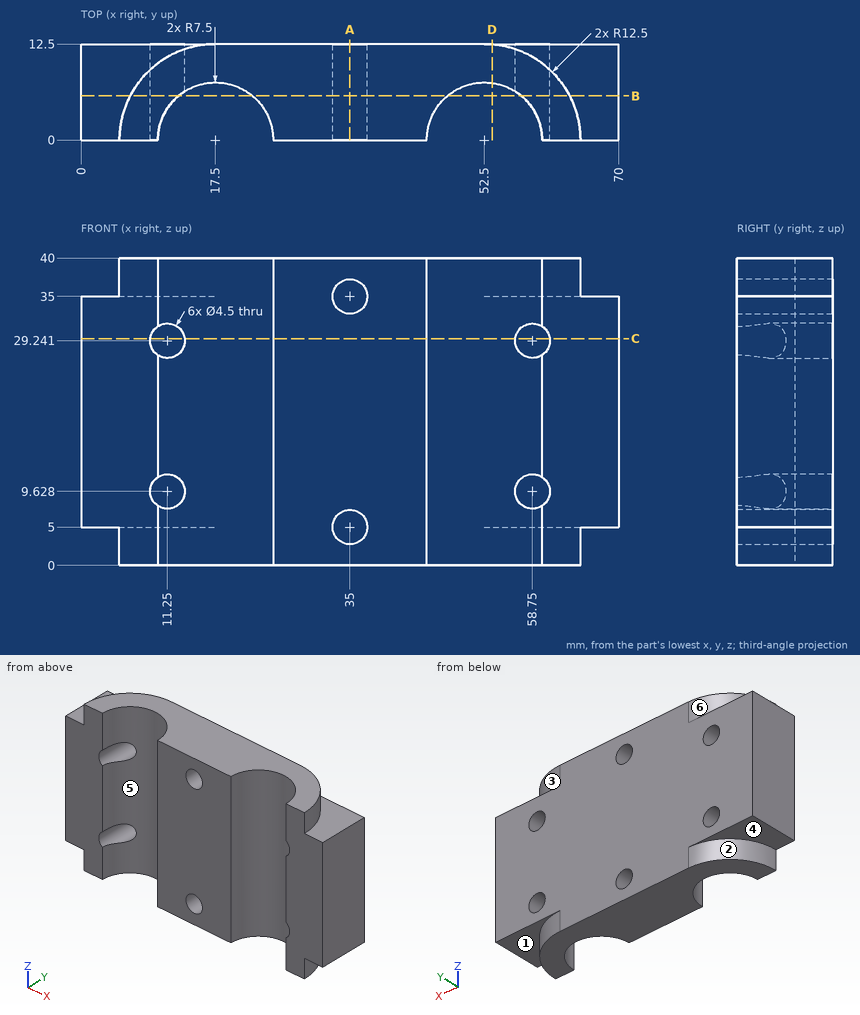
Check sheet for the drawn part. Datum: minimum x, y, z corner. Units: mm. A direction names the side the tool comes from. Give positions to 0.01 mm unless a question says otherwise; leave off trailing zeros. Loops run counter-clockwise (first coordinate to the right, second up) from the corner with the lowest first, then second, coordinate; pieces in that order, holes last.
1) Thickness scan on line 1 along Z through (x, y) = (11.25, 4.5); line 2 along X through (y, z) = (6, 17); line 3 along X through (y, z) = (1.5, 8.5). Record the ranges inside material, lowest first.
2) Set-up check for the marked faces 1, 2 and 3: record each of +Z, -Z, +X, -X, +Y, -Y from which the full face is reachable in a straight line by a thin tool's end or side.
3) Depth check by flat-ended pin: pin 1 Ø4 at (x, z) = (35, 5) entering from +Y. Enter the tip coordinate at first touch or a pass-through.
4) Sectioned sample at C-C, the plane z = 29.5. Enter the section's corners in (x, y) (1 decimal).
5) Sectioned sample at A-A, the plane x = 35. Enter the section's corners in (y, z).
6) Draft check along X on the marked faces 4, 5 and 6. Enter one of: pulls with the +X half, pulls with the -X half, needs draft (parallel to the pull), parting line crosses it, or undercut.
7) Sectioned sample at B-B, the plane y = 5.75. Count the separate pieces of the cut face and the enclosed holes in it, then the cut area to 3 significant figures.
8) Sectioned sample at D-D, the plane x = 53.5. Enter the section's corners in (y, z), then the cut area to 3 significant figures.
Answers:
1. line 1: z = 0 to 7.38, 11.88 to 26.99, 31.49 to 40
1. line 2: x = 0 to 13, 22 to 48, 57 to 70
1. line 3: x = 0 to 9.3, 24.85 to 45.15, 60.7 to 70
2. face 1: -Z, +X, +Y
2. face 2: -Z, -X, +Y
2. face 3: +Z, +X, +Y
3. pin 1: passes through
4. outline: (0, 0) - (9, 0) - (9, 12.5) - (0, 12.5) - close; (13.5, 6.3) arc R7.5 cw to (25, 0) - (45, 0) arc R7.5 cw to (56.5, 6.3) - (56.5, 12.5) - (13.5, 12.5) - close; (61, 0) - (70, 0) - (70, 12.5) - (61, 12.5) - close
5. outline: (0, 0) - (12.5, 0) - (12.5, 2.75) - (0, 2.75) - close; (0, 7.25) - (12.5, 7.25) - (12.5, 32.75) - (0, 32.75) - close; (0, 37.25) - (12.5, 37.25) - (12.5, 40) - (0, 40) - close
6. face 4: needs draft
6. face 5: undercut
6. face 6: pulls with the -X half
7. separate pieces: 3
7. enclosed holes: 2
7. area: 1,810 mm2
8. outline: (7.43, 0) - (12.46, 0) - (12.46, 5) - (12.5, 5) - (12.5, 35) - (12.46, 35) - (12.46, 40) - (7.43, 40) - close
8. area: 202 mm2
